```python
from build123d import *

# Parameters (mm, degrees)
SKETCH1_W               = 76.2
SKETCH1_H               = 25.4
BOSS_EXTRUDE1_DEPTH     = 9.525
CUT_EXTRUDE2_DEPTH      = 4.445
SKETCH2_R               = 1.905
CUT_EXTRUDE1_DEPTH      = 42.275
SKETCH5_R               = 2.032
CUT_EXTRUDE3_DEPTH      = 28.575
MIRROR2_COPY_1_SKETCH_R = 1.905
MIRROR2_COPY_1_DEPTH    = 42.275


with BuildPart() as part:
    # Sketch1 → Boss-Extrude1 (new body)
    with BuildSketch(Plane.XY):
        Rectangle(SKETCH1_W, SKETCH1_H)
    extrude(amount=BOSS_EXTRUDE1_DEPTH)

    # Sketch4 → Cut-Extrude2 (cut, symmetric)
    with BuildSketch(Plane(origin=(0, 0, 0), x_dir=(1, 0, 0), z_dir=(0, 1, 0))):
        with BuildLine():
            Line((-28.92425, -6.6675), (-28.92425, -9.525))
            Line((-28.92425, -9.525), (-18.76425, -9.525))
            Line((-18.76425, -9.525), (-18.76425, -6.6675))
            ThreePointArc((-18.76425, -6.6675), (-23.84425, -1.5875), (-28.92425, -6.6675))
        make_face()
    cut_extrude2 = extrude(amount=CUT_EXTRUDE2_DEPTH, both=True, mode=Mode.SUBTRACT)

    # Sketch2 → Cut-Extrude1 (cut, through all)
    with BuildSketch(Plane.XY.offset(9.525)):
        with Locations((-31.75, 7.9375)):
            Circle(SKETCH2_R)
    cut_extrude1 = extrude(amount=-CUT_EXTRUDE1_DEPTH, mode=Mode.SUBTRACT)

    # Sketch5 → Cut-Extrude3 (cut)
    with BuildSketch(Plane(origin=(0, 12.7, 0), x_dir=(1, 0, 0), z_dir=(0, 1, 0))):
        with Locations(Location((-23.84425, -6.6675, 0), (0, 0, 270))):
            Circle(SKETCH5_R)
    cut_extrude3 = extrude(amount=-CUT_EXTRUDE3_DEPTH, mode=Mode.SUBTRACT)

    # Mirror1: Cut-Extrude1 across plane
    add(cut_extrude1.mirror(Plane.ZX), mode=Mode.SUBTRACT)

    # Mirror2: Cut-Extrude2, Cut-Extrude1, Cut-Extrude3 across plane
    add(cut_extrude2.mirror(Plane.ZY.offset(12.7)), mode=Mode.SUBTRACT)
    add(cut_extrude1.mirror(Plane.ZY.offset(12.7)), mode=Mode.SUBTRACT)
    add(cut_extrude3.mirror(Plane.ZY.offset(12.7)), mode=Mode.SUBTRACT)

    # Mirror2 copy 1 sketch → Mirror2 copy 1 (cut, through all)
    with BuildSketch(Plane(origin=(-25.4, 0, 9.525), x_dir=(-1, 0, 0), z_dir=(0, 0, 1))):
        with Locations((-31.75, 7.9375)):
            Circle(MIRROR2_COPY_1_SKETCH_R)
    extrude(amount=-MIRROR2_COPY_1_DEPTH, mode=Mode.SUBTRACT)


solid = part.part
```
Can you work these out from the model? Positions are in its coordinate system, mm. A direction names the side the tool comes from. Round coordinates to 2 decimals unless told otherwise and drop trailing zeros. Loops run counter-clockwise (first coordinate to the right, second up) from the corner with the lowest first, then second, coordinate; pieces in that order, holes last. Notation, with made-up numbers: (51.5, 17) -> (72.5, 17) arc R5 cw to (72.5, 23) -> close; hole circle Ø11 at (75, 59). An arc over 180 degrees is marked (long way). One line per item, written item: value. Start each with the question number.
1. If we section it at C-C, the plane x = -31.75: Write out the boundary of the cut face in (y, z) (1 decimal).
2. If I drill on probe 1 along X at (y, z) = (2.5, 8.5); probe 2 along Y at (x, z) = (-31.75, 3.5); probe 3 along Y at (x, z) = (-21, 8.5) (3 decimals), over which ranges is the centre line in solid material (lowest first)?
3. For faces 5 (the cylindrical face through (-33.154, -9.225, 4.829)), 6 (the cylindrical face through (-23.73, 0.06, 1.59)), which set-ups out of +Z, -Z, +X, -X, +Y, -Y let a thin tool reach every point of the face, with its end or its side?
4. If we section it at B-B, the plane y = -9: Write out the boundary of the cut face in (x, z) (1 decimal), then the cut area to 3 significant figures.
5. For pin 1 (2.5 mm diameter, centred on x = -23.84, z = 6.67, fed in from -Y), with a flat end and sliding along its axis, tell me the tip position at first contact or that it passes through.
6. If we mould it in two halves opening along X, with no side actions, what happens to faces 1 (the flat face through (-0.5, 12.7, 4.7)), 2 (the flat face through (-38.1, 0, 5)), 3 (the cylindrical face through (-1.67, 0.06, 1.59)), 4 (the cylindrical face through (7.754, 9.225, 4.829))? For each: pulls with the +X half, pulls with the -X half, needs draft (parallel to the pull), parting line crosses it, or undercut.
7. If we section it at D-D, the plane y = 2: Write out the boundary of the cut face in (x, z) (1 decimal).
8. If we section it at A-A, the plane z = 6: Give the number of separate pieces and of enclosed holes in the cut face, then the cut area to 3 significant figures.
Calculated:
1. outline: (-12.7, 0) -> (-9.8, 0) -> (-9.8, 9.5) -> (-12.7, 9.5) -> close; (-6, 0) -> (6, 0) -> (6, 9.5) -> (-6, 9.5) -> close; (9.8, 0) -> (12.7, 0) -> (12.7, 9.5) -> (9.8, 9.5) -> close
2. probe 1: x = -38.1 to -28.92, -18.76 to -6.64, 3.52 to 38.1
2. probe 2: y = -12.7 to -9.84, -6.03 to 6.03, 9.84 to 12.7
2. probe 3: y = -12.7 to -4.445, 4.445 to 12.7
3. face 5: +Z, -Z
3. face 6: +Z
4. outline: (-38.1, 0) -> (-33.3, 0) -> (-33.3, 9.5) -> (-38.1, 9.5) -> close; (-30.2, 0) -> (4.8, 0) -> (4.8, 9.5) -> (-30.2, 9.5) -> close; (7.9, 0) -> (38.1, 0) -> (38.1, 9.5) -> (7.9, 9.5) -> close; hole circle Ø4.1 at (-23.8, 6.7); hole circle Ø4.1 at (-1.6, 6.7)
4. area: 640 mm²
5. pin 1: passes through
6. face 1: needs draft
6. face 2: pulls with the -X half
6. face 3: undercut
6. face 4: undercut
7. outline: (-38.1, 0) -> (38.1, 0) -> (38.1, 9.5) -> (3.5, 9.5) -> (3.5, 6.7) arc R5.1 cw to (-6.6, 6.7) -> (-6.6, 9.5) -> (-18.8, 9.5) -> (-18.8, 6.7) arc R5.1 cw to (-28.9, 6.7) -> (-28.9, 9.5) -> (-38.1, 9.5) -> close
8. separate pieces: 3
8. enclosed holes: 4
8. area: 1,580 mm²
